The figure shows three views and two pictorial views of one solid part (mm, origin at its lowest corner). Answer the questions. A direction names the side the tool comes from. Coordinates: 2 decimals unless noted, no trailing zeros. Order: outer loops, then holes, each group sorted by start corner. A loop starts at its lowest first (then second) coordinate and runs counter-clockwise, first axis right, second up. Notation, with made-up numbers: (-36, 35) -> (-8, 35) arc R31 cw to (-8, 72) -> close; hole circle Ø6 at (-28, -23). An arc over 180 degrees is marked (long way). Return JSON: item names as keys, results as strings.
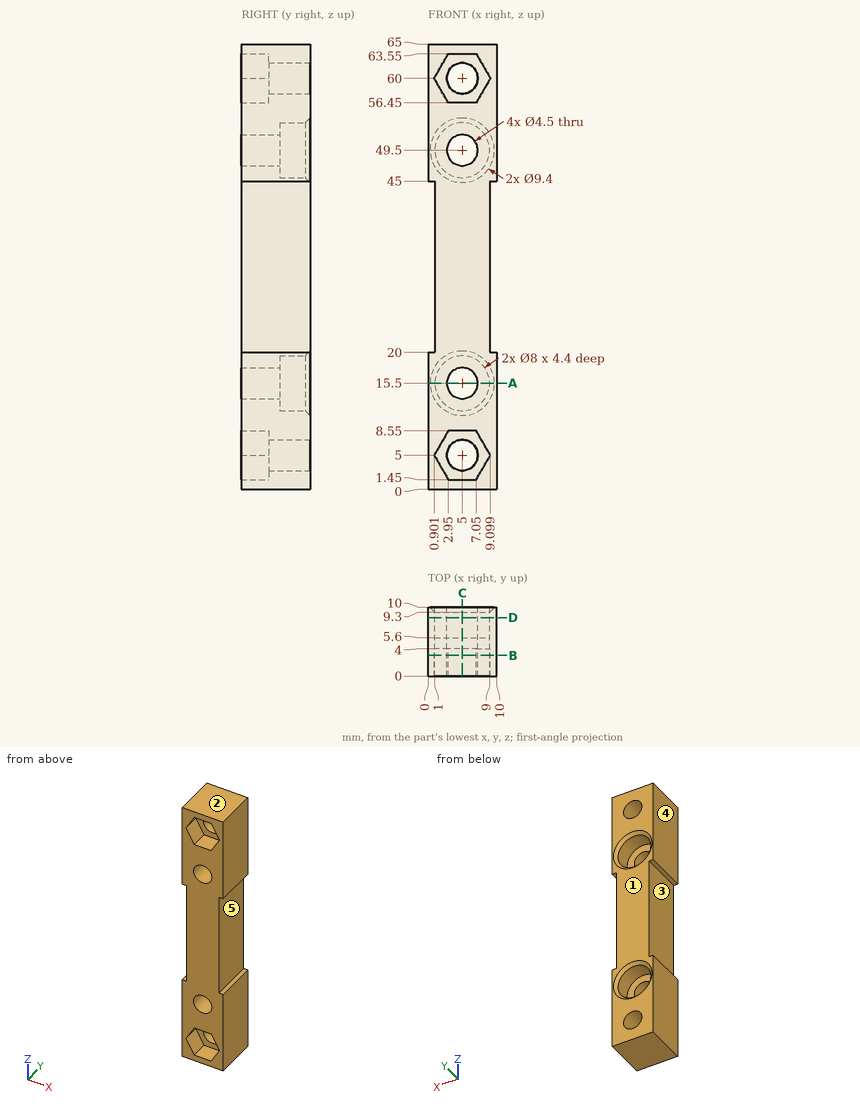
1. The part is cut by section C-C on x = 5. Give the number of separate pieces and of enclosed holes in the cut face.
Answer block:
{"separate pieces": "5", "enclosed holes": "0"}
2. Consider line 1 (Z direction, x = 5, y = 7.1); line 2 (Z direction, x = 5, y = 5.5); line 3 (Z direction, x = 8, y = 6) (1 decimal). Determine where each line is inside the solid, lowest interval first. Write a range as from..to.
Answer block:
{"line 1": "z = 0..2.75, 7.25..11.5, 19.5..45.5, 53.5..57.75, 62.25..65", "line 2": "z = 0..2.75, 7.25..13.25, 17.75..47.25, 51.75..57.75, 62.25..65", "line 3": "z = 0..12.9, 18.1..46.9, 52.1..65"}
3. For the marked faces 4 and 5, determine the directions among +Z, -Z, +X, -X, +Y, -Y from which every point of the face is accessible in a straight line to the end or side of a thin tool.
Answer block:
{"face 4": "+Z, -Z, -X, +Y, -Y", "face 5": "+X, +Y, -Y"}
4. The part is cut by section A-A on z = 15.5. Give the vertices of the cut face in (x, y).
Answer block:
{"outline": "(0, 0) -> (2.75, 0) -> (2.75, 5.6) -> (1, 5.6) -> (1, 9.3) -> (0.3, 10) -> (0, 10) -> close; (7.25, 0) -> (10, 0) -> (10, 10) -> (9.7, 10) -> (9, 9.3) -> (9, 5.6) -> (7.25, 5.6) -> close"}
5. Determine the mould class of the marked faces 1, 2 and 3 for opening direction Z: pulls with the +Z half, pulls with the -Z half, needs draft (parallel to the pull), parting line crosses it, or undercut.
Answer block:
{"face 1": "needs draft", "face 2": "pulls with the +Z half", "face 3": "undercut"}
6. This flat-tipped pin is pushed along its axis until it touches: pin 1 Ø2 at (x, z) = (5.5, 6.5) entering from -Y. Where does it stop, or does it pass through?
Answer block:
{"pin 1": "stops at y = 4"}
7. The part is cut by section B-B on y = 3. Give the vertices of the cut face in (x, z), and give its area (3 significant figures).
Answer block:
{"outline": "(0, 0) -> (10, 0) -> (10, 20) -> (9, 20) -> (9, 45) -> (10, 45) -> (10, 65) -> (0, 65) -> (0, 45) -> (1, 45) -> (1, 20) -> (0, 20) -> close; hole (0.9, 5) -> (2.95, 1.45) -> (7.05, 1.45) -> (9.1, 5) -> (7.05, 8.55) -> (2.95, 8.55) -> close; hole (0.9, 60) -> (2.95, 56.45) -> (7.05, 56.45) -> (9.1, 60) -> (7.05, 63.55) -> (2.95, 63.55) -> close; hole circle Ø4.5 at (5, 15.5); hole circle Ø4.5 at (5, 49.5)", "area": "481 mm2"}
8. The part is cut by section D-D on y = 8.5. Give the vertices of the cut face in (x, z).
Answer block:
{"outline": "(0, 0) -> (10, 0) -> (10, 20) -> (9, 20) -> (9, 45) -> (10, 45) -> (10, 65) -> (0, 65) -> (0, 45) -> (1, 45) -> (1, 20) -> (0, 20) -> close; hole circle Ø8 at (5, 15.5); hole circle Ø8 at (5, 49.5); hole circle Ø4.5 at (5, 5); hole circle Ø4.5 at (5, 60)"}
